```python
from build123d import *

# Parameters (mm, degrees)
SKETCH2_R               = 2.5
CUT_EXTRUDE3_DEPTH      = 91.495856259
CUT_EXTRUDE6_DEPTH      = 92.681513949
CUT_EXTRUDE6_DEPTH_BACK = 92.681513949
SKETCH6_R               = 2.5


with BuildPart() as part:
    # Sketch1 → Revolve1 (revolve)
    with BuildSketch(Plane.XY, mode=Mode.PRIVATE) as revolve1_sk:
        Polygon((-41.5, -29), (-41.5, -4), (-61.5, -4), (-61.5, 0), (-37.5, 0), (-37.5, -4), (-33.5, -4), (-33.5, -15), (-37.5, -15), (-37.5, -29), align=None)
    revolve(revolve1_sk.sketch.rotate(Axis((0, -100.5, 0), (0, 1, 0)), 270), axis=Axis((0, -100.5, 0), (0, 1, 0)))

    # Sketch2 → Cut-Extrude3 (cut, through all)
    with BuildSketch(Plane.XZ.offset(4)):
        with Locations(Location((55, 0, 0), (0, 0, 270))):
            Circle(SKETCH2_R)
        with Locations(Location((-55, 0, 0), (0, 0, 270))):
            Circle(SKETCH2_R)
        with Locations(Location((0, 55, 0), (0, 0, 270))):
            Circle(SKETCH2_R)
        with Locations(Location((0, -55, 0), (0, 0, 270))):
            Circle(SKETCH2_R)
    extrude(amount=-CUT_EXTRUDE3_DEPTH, mode=Mode.SUBTRACT)

    # Sketch6 → Cut-Extrude6 (cut, two sides: drawn at the far end of the back side and taken through both)
    with BuildSketch(Plane.XY.offset(-CUT_EXTRUDE6_DEPTH_BACK)):
        with Locations((0, -19)):
            Circle(SKETCH6_R)
    extrude(amount=CUT_EXTRUDE6_DEPTH + CUT_EXTRUDE6_DEPTH_BACK, mode=Mode.SUBTRACT)


solid = part.part
```
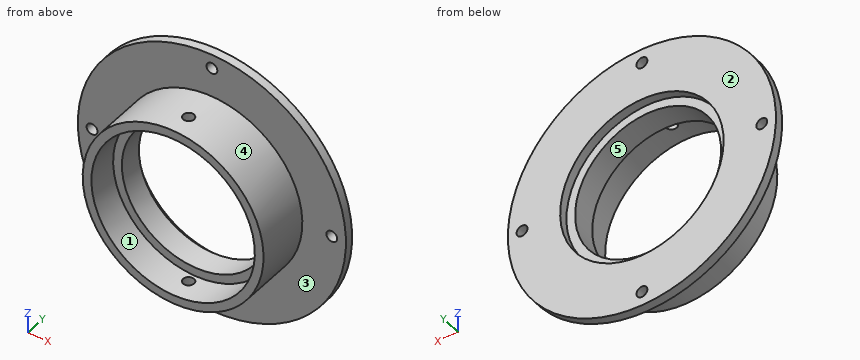
Here's how the part is built. I have some questions about the finished solid (model axes, mm). Face numbers are marked on the shaded views. A direction names the side the tool comes from. Round coordinates to 2 decimals unless told otherwise and drop trailing zeros. Order: outer loops, then holes, each group sorted by start corner. A loop starts at its lowest first (then second) coordinate and runs counter-clockwise, first axis right, second up. Notation, with made-up numbers: (-40, -24) -> (-15, -24) arc R24 cw to (-15, 11) -> close; hole circle Ø4 at (4, 52). An arc over 180 degrees is marked (long way). Use a Markdown table: item, result. Add a question column.
(1) For the marked faces 1 and 2, which set-ups out of +Z, -Z, +X, -X, +Y, -Y let a thin tool reach every point of the face, with its end or its side?
(2) For pin 1 Ø1 at (y, z) = (-16, -1) entering from +X; pin 2 Ø6 at (x, z) = (45.5, -4.5) entering from -Y; pin 3 Ø10 at (y, z) = (-16.5, -13) entering from -X; pin 4 Ø4.5 at (x, z) = (55, 0) entering from +Y, each with a flat end and sliding along its axis, tell me the tip position at first contact or that it passes through.
(3) Suppose I cut it at C-C, the plane z = -13. Please give me the cut outline in (x, y).
(4) If we mould it in two halves opening along Z, with no side actions, what happens to the marked faces 3, 4 and 5? For each: released by +Z, released by -Z, zero draft, split by the parting line, or undercut.
(5) Suppose I cut it at B-B, the plane x = 24.5. Please give me the cut outline in (y, z), and give its area (3 significant figures).
(6) Suppose I cut it at D-D, the plane y = -24.5. Please give me the cut outline in (x, z), and give its area (3 significant figures).
(7) Suppose I cut it at A-A, the plane z = 0. Please give me the cut outline in (x, y).
(8) I need wall thicknesses on line 1 along X through (y, z) = (-1.35, 0); line 2 along Z through (x, y) = (-0.5, -25.5); line 3 along Y through (x, z) = (-44.5, -17.5). Which ranges of each line are inside material? Lowest first, please.
Verdict:
| question | item | result |
|---|---|---|
| 1 | face 1 | -Y |
| 1 | face 2 | +Z, -Z, +X, -X, +Y |
| 2 | pin 1 | x = 41.5 |
| 2 | pin 2 | y = -4 |
| 2 | pin 3 | x = -40.72 |
| 2 | pin 4 | through |
| 3 | outline | (-60.11, -4) -> (-39.41, -4) -> (-39.41, -29) -> (-35.17, -29) -> (-35.17, -15) -> (-30.87, -15) -> (-30.87, -4) -> (-35.17, -4) -> (-35.17, 0) -> (-60.11, 0) -> close; (30.87, -15) -> (35.17, -15) -> (35.17, -29) -> (39.41, -29) -> (39.41, -4) -> (60.11, -4) -> (60.11, 0) -> (35.17, 0) -> (35.17, -4) -> (30.87, -4) -> close |
| 4 | face 3 | zero draft |
| 4 | face 4 | split by the parting line |
| 4 | face 5 | undercut |
| 5 | outline | (-29, -33.5) -> (-4, -33.5) -> (-4, -56.41) -> (0, -56.41) -> (0, -28.39) -> (-4, -28.39) -> (-4, -22.85) -> (-15, -22.85) -> (-15, -28.39) -> (-29, -28.39) -> close; (-29, 28.39) -> (-15, 28.39) -> (-15, 22.85) -> (-4, 22.85) -> (-4, 28.39) -> (0, 28.39) -> (0, 56.41) -> (-4, 56.41) -> (-4, 33.5) -> (-29, 33.5) -> close |
| 5 | area | 601 mm2 |
| 6 | outline | circle Ø83 at (0, 0); hole circle Ø75 at (0, 0) |
| 6 | area | 993 mm2 |
| 7 | outline | (-61.5, -4) -> (-57.5, -4) -> (-57.5, 0) -> (-61.5, 0) -> close; (-52.5, -4) -> (-41.5, -4) -> (-41.5, -29) -> (-37.5, -29) -> (-37.5, -15) -> (-33.5, -15) -> (-33.5, -4) -> (-37.5, -4) -> (-37.5, 0) -> (-52.5, 0) -> close; (33.5, -15) -> (37.5, -15) -> (37.5, -29) -> (41.5, -29) -> (41.5, -4) -> (52.5, -4) -> (52.5, 0) -> (37.5, 0) -> (37.5, -4) -> (33.5, -4) -> close; (57.5, -4) -> (61.5, -4) -> (61.5, 0) -> (57.5, 0) -> close |
| 8 | line 1 | -61.5 to -57.5, -52.5 to -37.5, 37.5 to 52.5, 57.5 to 61.5 |
| 8 | line 2 | -41.5 to -37.5, 37.5 to 41.5 |
| 8 | line 3 | -4 to 0 |
